CAD build for the part. Positions are in the model's coordinates, mm. Face numbers are marked on the shaded views. A direction names the side the tool comes from. Give positions to 0.01 mm unless a question says otherwise; leave off trailing zeros. Write each loop counter-clockwise with the first axis right and the second up, starting at its lowest first coordinate (ties: lowest second). Pieces come first, ordered by that corner, then holes. Notation, with made-up numbers: (86.25, -10) - (104.25, -10) arc R20 cw to (104.25, 1) - close; hole circle Ø4 at (40.25, -29). An arc over 180 degrees is marked (long way). Answer as a JSON object with one key per item and string values.
Autodesk Fusion 360 part; units mm, degrees
sketch "Sketch1" plane through (0, 0, 0) normal (0, 0, 1) x (1, 0, 0)
  circle A0 centre (0, 0) radius 3.5
  dimension "d1" = 7
extrude "Extrude1" add sketch "Sketch1" along normal blind 6
sketch "Sketch2" plane through (0, 0, 0) normal (0, 0, 1) x (1, 0, 0)
  line L0 (0, 3.25) -> (13.701, 3.25)
  line L1 (13.701, 3.25) -> (13.701, -3.25)
  line L2 (13.701, -3.25) -> (0, -3.25)
  line L3 (0, -3.25) -> (0, 3.25)
  dimension "d4" = 6.5
  dimension "d5" = 13.701
extrude "Extrude2" add sketch "Sketch2" along normal blind 2
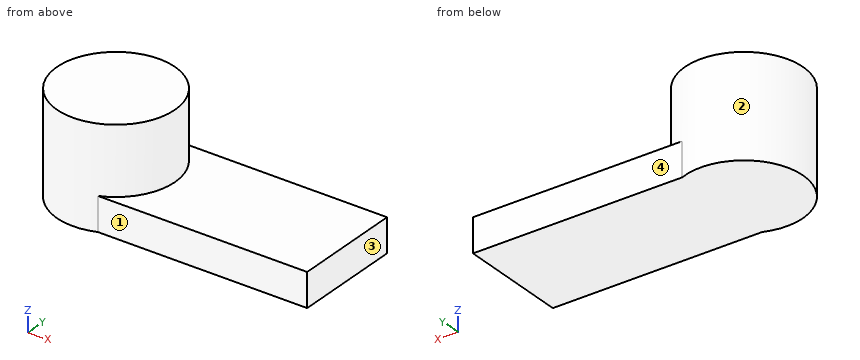
Item 1: Cut at D-D (x = 2.25). Give the cut face in (y, z), and give its area (3 significant figures).
Entries:
{"outline": "(-3.25, 0) - (3.25, 0) - (3.25, 2) - (2.68, 2) - (2.68, 6) - (-2.68, 6) - (-2.68, 2) - (-3.25, 2) - close", "area": "34.4 mm2"}
Item 2: Which spindle directions (+Z, -Z, +X, -X, +Y, -Y) get a long thin tool onto all of the face, cutting with end or side? Do the marked faces 1, 2, 3 and 4. Say none if no direction does.
Entries:
{"face 1": "+Z, -Z, +X, -Y", "face 2": "+Z", "face 3": "+Z, -Z, +X, +Y, -Y", "face 4": "+Z, -Z, +X, +Y"}
Item 3: Cut at C-C (x = 10.25). Give the cut face in (y, z).
Entries:
{"outline": "(-3.25, 0) - (3.25, 0) - (3.25, 2) - (-3.25, 2) - close"}
Item 4: Cut at B-B (z = 0.7). Give the cut face in (x, y).
Entries:
{"outline": "(1.3, -3.25) - (13.7, -3.25) - (13.7, 3.25) - (1.3, 3.25) arc R3.5 ccw (long way) to start"}
Item 5: Probe line 1 (Z direction, x = 7, y = -0.75); line 2 (Y direction, x = 9.25, z = 0.55); line 3 (X direction, y = 0, z = 3.65). List the from-to ranges inside material, lowest first. Write a range as from..to.
Entries:
{"line 1": "0..2", "line 2": "-3.25..3.25", "line 3": "-3.5..3.5"}
Item 6: Cut at A-A (y = 0). Give the cut face in (x, z), and give its area (3 significant figures).
Entries:
{"outline": "(-3.5, 0) - (13.7, 0) - (13.7, 2) - (3.5, 2) - (3.5, 6) - (-3.5, 6) - close", "area": "62.4 mm2"}
Item 7: Flat gauge pins, fed straight in: P1, Ø0.6, axis at x = 8, z = 1, coming from the +Y side; P2, Ø1.5, axis at x = 9, z = 1.5, coming from the -Y side. Where does each tip first touch, or does it go through?
Entries:
{"P1": "y = 3.25", "P2": "y = -3.25"}
